The model under review builds one solid part; all positions refer to its coordinate system, in mm. Face numbers are marked on the shaded views. Give positions to 0.01 mm unless a question says otherwise; leave off trailing zeros. Loops run counter-clockwise (first coordinate to the right, second up) from the corner with the lowest first, then second, coordinate; pieces in that order, holes last. Notation, with made-up numbers: (67, -32) - (103, -32) arc R27 ccw to (103, 4) - close; hole circle Ø2 at (40, -9). An arc over 180 degrees is marked (long way). Answer as a JSON object with one key per item and string values.
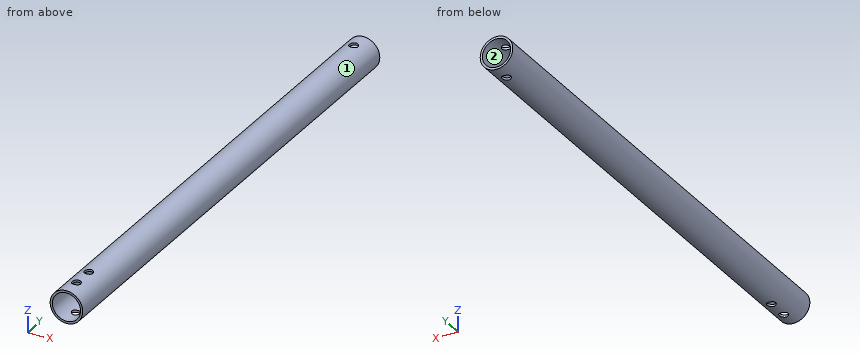
from build123d import *

# Parameters (mm, degrees)
SKETCH1_R           = 7.5
SKETCH1_R_2         = 6.5
BOSS_EXTRUDE1_DEPTH = 240
SKETCH2_R           = 2
CUT_EXTRUDE1_DEPTH  = 9


with BuildPart() as part:
    # Sketch1 → Boss-Extrude1 (new body)
    with BuildSketch(Plane(origin=(0, 0, 0), x_dir=(1, 0, 0), z_dir=(0, 1, 0))):
        Circle(SKETCH1_R)
        Circle(SKETCH1_R_2, mode=Mode.SUBTRACT)
    extrude(amount=BOSS_EXTRUDE1_DEPTH)

    # Sketch2 → Cut-Extrude1 (cut, symmetric)
    with BuildSketch(Plane.XY):
        with Locations((0, 8)):
            Circle(SKETCH2_R)
        with Locations((0, 18)):
            Circle(SKETCH2_R)
        with Locations((0, 242)):
            Circle(SKETCH2_R)
        with Locations((0, 232)):
            Circle(SKETCH2_R)
    extrude(amount=CUT_EXTRUDE1_DEPTH, both=True, mode=Mode.SUBTRACT)


solid = part.part
Q1. The part is to be moulded in two halves that separate along X. For the marked faces 1 and 2, say which applies: +X half, -X half, draft (parallel to the pull), parting line (faces both ways), or undercut.
Results:
{"face 1": "parting line", "face 2": "undercut"}
Q2. Consider section D-D, the plane y = 50. State the section outline as (x, z) points.
Results:
{"outline": "circle Ø15 at (0, 0); hole circle Ø13 at (0, 0)"}
Q3. Consider section B-B, the plane z = 0. State the section outline as (x, y) points, plus the area to 3 significant figures.
Results:
{"outline": "(-7.5, 0) - (-6.5, 0) - (-6.5, 240) - (-7.5, 240) - close; (6.5, 0) - (7.5, 0) - (7.5, 240) - (6.5, 240) - close", "area": "480 mm^2"}
Q4. Consider section C-C, the plane y = 232. State the section outline as (x, z) points, plus the area to 3 significant figures.
Results:
{"outline": "(-2, -7.23) - (-2, -6.18) arc R6.5 cw to (-2, 6.18) - (-2, 7.23) arc R7.5 ccw to start; (2, -7.23) arc R7.5 ccw to (2, 7.23) - (2, 6.18) arc R6.5 cw to (2, -6.18) - close", "area": "35.9 mm^2"}
Q5. To check wall thickness, follow probe 1 along Y at (x, z) = (0, 7.1); probe 2 along X at (y, z) = (36.5, 0); probe 3 along Z at (x, y) = (5, 125.5). State the ranges of each line that lie inside material, in increasing order. Write a range as [from, to].
Results:
{"probe 1": "y = [0, 6], [10, 16], [20, 230], [234, 240]", "probe 2": "x = [-7.5, -6.5], [6.5, 7.5]", "probe 3": "z = [-5.59, -4.15], [4.15, 5.59]"}
Q6. Clearance check with flat-ended pins moving along their axes: pin 1 Ø8 at (x, z) = (0, 0) entering from +Y; pin 2 Ø3 at (x, y) = (4.5, 33) entering from -Z; pin 3 Ø5 at (x, y) = (-3, 199.5) entering from +Z; pin 4 Ø2 at (x, y) = (-2, 104.5) entering from +Z. State where each tip first meets the part, or that it passes through.
Results:
{"pin 1": "passes through", "pin 2": "stops at z = -6.87", "pin 3": "stops at z = 7.48", "pin 4": "stops at z = 7.43"}
Q7. Consider section A-A, the plane x = 0. State how many separate pieces and enclosed holes the cut face has, plus the area to 3 significant figures.
Results:
{"separate pieces": "8", "enclosed holes": "0", "area": "456 mm^2"}
